Geometry check sheet. Reference: drawing and pictorial views, mm from the part's lowest x, y, z. A direction names the side the tool comes from. Coordinates: 2 decimals unless noted, no trailing zeros. Order: outer loops, then holes, each group sorted by start corner. A loop starts at its lowest first (then second) coordinate and runs counter-clockwise, first axis right, second up. Notation, with made-up numbers: (-15.5, 85.25) -> (28.5, 85.25) arc R15 cw to (28.5, 95.25) -> close; hole circle Ø1 at (12.5, -30). An arc over 180 degrees is marked (long way). Use CSV: the item, a comma, the result in double quotes. Start each with the question number.
1) Release check for a two-part mould opening along X. For the marked faces 3, 4 and 5 record: released by +X, released by -X, zero draft, split by the parting line, or undercut.
2) Sectioned sample at A-A on x = 10. Record the boundary of the cut face in (y, z), then the cut area to 3 significant figures.
3) Scan lines: line 1 along Z through (x, y) = (10, 3.8); line 2 along Z through (x, y) = (10, 2.3); line 3 along Y through (x, z) = (18.25, 6). Record each from-to range of solid material in increasing order.
4) Tool access check on the marked faces 1 and 2. Record the directions out of +Z, -Z, +X, -X, +Y, -Y that give a thin tool (end or side, any length) a straight path to the whole face; none if there is none.
5) Sectioned sample at C-C on y = 3.25. Record the boundary of the cut face in (x, z), then the cut area to 3 significant figures.
6) Sectioned sample at D-D on x = 3. Record the boundary of the cut face in (y, z).
7) Go/stop test with flat-tipped pins: pin 1 (3 mm diameter, centred on x = 9.5, z = 9, fed in from -Y); pin 2 (2.5 mm diameter, centred on x = 10, z = 17, fed in from +Y); pin 3 (2 mm diameter, centred on y = 1, z = 7, fed in from -X); pin 4 (2 mm diameter, centred on x = 15.5, z = 14, fed in from -Y). Record where each tip stops, or that it passes through.
8) Sectioned sample at B-B on z = 10. Record the boundary of the cut face in (x, y).
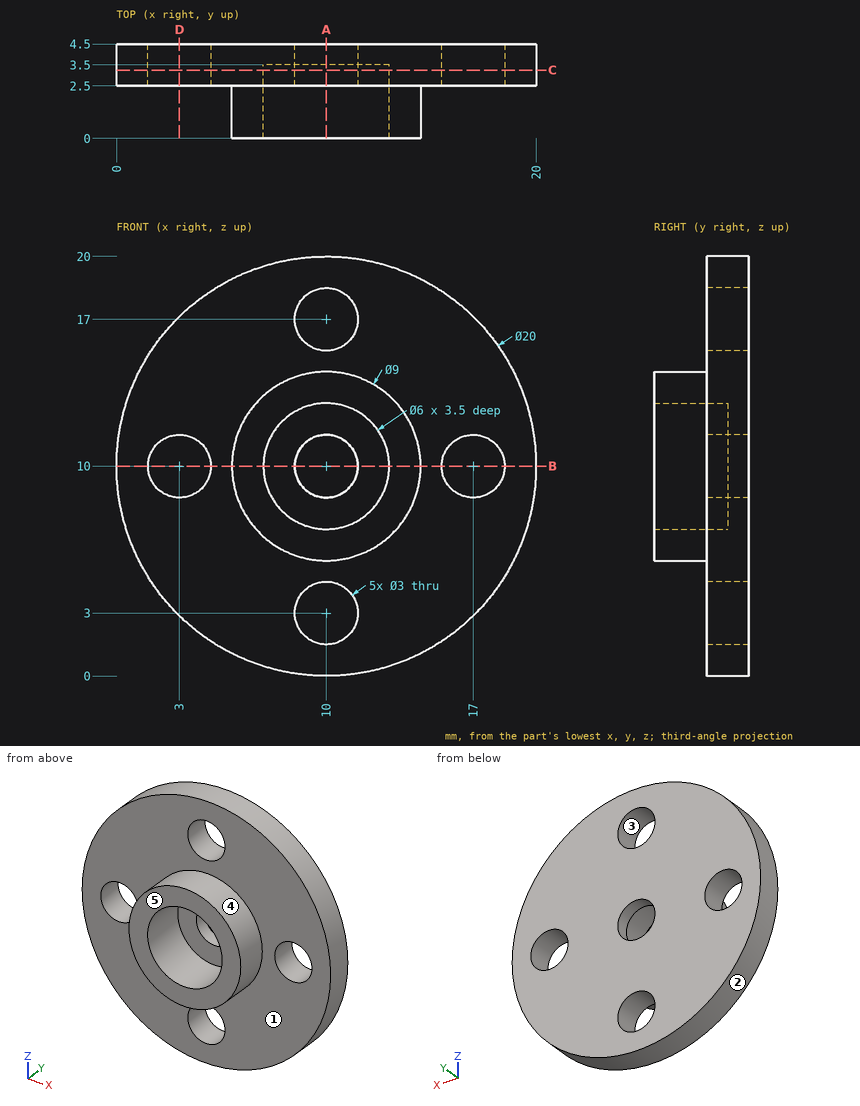
Answers follow:
1,face 3,"undercut"
1,face 4,"split by the parting line"
1,face 5,"zero draft"
2,outline,"(0, 5.5) -> (2.5, 5.5) -> (2.5, 4.5) -> (4.5, 4.5) -> (4.5, 8.5) -> (3.5, 8.5) -> (3.5, 7) -> (0, 7) -> close; (0, 13) -> (3.5, 13) -> (3.5, 11.5) -> (4.5, 11.5) -> (4.5, 15.5) -> (2.5, 15.5) -> (2.5, 14.5) -> (0, 14.5) -> close; (2.5, 0) -> (4.5, 0) -> (4.5, 1.5) -> (2.5, 1.5) -> close; (2.5, 18.5) -> (4.5, 18.5) -> (4.5, 20) -> (2.5, 20) -> close"
2,area,"26.5 mm²"
3,line 1,"z = 0 to 1.5, 4.5 to 8.5, 11.5 to 15.5, 18.5 to 20"
3,line 2,"z = 5.5 to 7, 13 to 14.5"
3,line 3,"y = 2.5 to 4.5"
4,face 1,"-Y"
4,face 2,"+Y, -Y"
5,outline,"circle Ø20 at (10, 10); hole circle Ø3 at (3, 10); hole circle Ø6 at (10, 10); hole circle Ø3 at (10, 3); hole circle Ø3 at (10, 17); hole circle Ø3 at (17, 10)"
5,area,"258 mm²"
6,outline,"(2.5, 2.86) -> (4.5, 2.86) -> (4.5, 8.5) -> (2.5, 8.5) -> close; (2.5, 11.5) -> (4.5, 11.5) -> (4.5, 17.14) -> (2.5, 17.14) -> close"
7,pin 1,"stops at y = 3.5"
7,pin 2,"passes through"
7,pin 3,"stops at x = 5.97"
7,pin 4,"stops at y = 2.5"
8,outline,"(0, 2.5) -> (1.5, 2.5) -> (1.5, 4.5) -> (0, 4.5) -> close; (4.5, 2.5) -> (5.5, 2.5) -> (5.5, 0) -> (7, 0) -> (7, 3.5) -> (8.5, 3.5) -> (8.5, 4.5) -> (4.5, 4.5) -> close; (11.5, 3.5) -> (13, 3.5) -> (13, 0) -> (14.5, 0) -> (14.5, 2.5) -> (15.5, 2.5) -> (15.5, 4.5) -> (11.5, 4.5) -> close; (18.5, 2.5) -> (20, 2.5) -> (20, 4.5) -> (18.5, 4.5) -> close"
